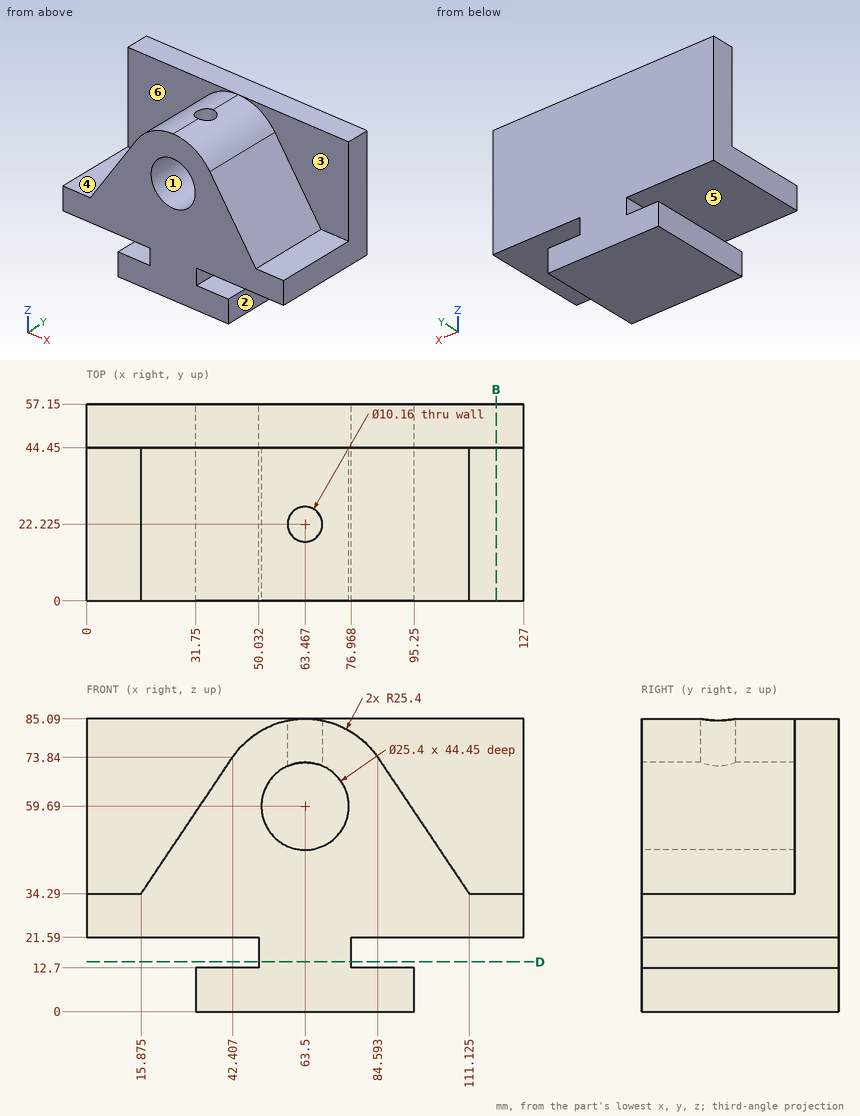
Here's the drawing with two shaded views (mm, measured from the low corner). I have some questions. A direction names the side the tool comes from. Round coordinates to 2 decimals unless told otherwise and drop trailing zeros. Order: outer loops, then holes, each group sorted by start corner. A loop starts at its lowest first (then second) coordinate and runs counter-clockwise, first axis right, second up. Notation, with made-up numbers: (-26, 13.25) -> (7, 13.25) arc R27 ccw to (7, 52.25) -> close; hole circle Ø2 at (42.25, 21). An arc over 180 degrees is marked (long way). Use a Markdown table: item, result. Add a question column.
(1) Suppose I cut it at D-D, the plane z = 14.5. Please give me the cut outline in (x, y), and give its area (3 significant figures).
(2) If we mould it in two halves opening along Z, with no side actions, what happens to the marked faces 4, 5 and 6? For each: released by +Z, released by -Z, zero draft, split by the parting line, or undercut.
(3) Suppose I cut it at B-B, the plane x = 119. Please give me the cut outline in (y, z), and give its area (3 significant figures).
(4) For the marked faces 1, 2 and 3, which set-ups out of +Z, -Z, +X, -X, +Y, -Y let a thin tool reach every point of the face, with its end or its side?
(5) I need wall thicknesses on line 1 along Z through (x, y) = (63.5, 27.5); line 2 along Y through (x, z) = (24, 81); line 3 along Z through (x, y) = (112.5, 35). Which ranges of each line are inside material? Lowest first, please.
(6) For pin 1 Ø12.5 at (x, z) = (58, 58) entering from -Y; pin 2 Ø6 at (y, z) = (32, 74.5) entering from +X; pin 3 Ø1 at (x, y) = (113, 11.5) entering from -Z; pin 4 Ø2 at (x, z) = (37, 20) entering from +Y, each with a flat end and sliding along its axis, tell me the tip position at first contact or that it passes through.
Verdict:
| question | item | result |
|---|---|---|
| 1 | outline | (50.03, 0) -> (76.97, 0) -> (76.97, 57.15) -> (50.03, 57.15) -> close |
| 1 | area | 1,540 mm2 |
| 2 | face 4 | released by +Z |
| 2 | face 5 | undercut |
| 2 | face 6 | zero draft |
| 3 | outline | (0, 21.59) -> (57.15, 21.59) -> (57.15, 85.09) -> (44.45, 85.09) -> (44.45, 34.29) -> (0, 34.29) -> close |
| 3 | area | 1,370 mm2 |
| 4 | face 1 | -Y |
| 4 | face 2 | -Z, +X, +Y, -Y |
| 4 | face 3 | +Z, +X, -Y |
| 5 | line 1 | 0 to 46.99, 72.39 to 85.09 |
| 5 | line 2 | 44.45 to 57.15 |
| 5 | line 3 | 21.59 to 34.29 |
| 6 | pin 1 | y = 44.45 |
| 6 | pin 2 | x = 86.16 |
| 6 | pin 3 | z = 21.59 |
| 6 | pin 4 | through |
